```python
from build123d import *

# Parameters (mm, degrees)
SKETCH1_W           = 190.5
SKETCH1_H           = 190.5
SKETCH1_R           = 1.905
SKETCH1_R_2         = 1.778
BOSS_EXTRUDE1_DEPTH = 6.35
BOSS_EXTRUDE3_DEPTH = 6.35
SKETCH8_R           = 3.175
CUT_EXTRUDE1_DEPTH  = 7.35
SKETCH9_R           = 3.175
CUT_EXTRUDE2_DEPTH  = 7.35
SKETCH10_R          = 1.5875
CUT_EXTRUDE3_DEPTH  = 7.35
SKETCH11_R          = 8.41375
CUT_EXTRUDE4_DEPTH  = 7.35


with BuildPart() as part:
    # Sketch1 → Boss-Extrude1 (new body)
    with BuildSketch(Plane(origin=(0, 0, 0), x_dir=(1, 0, 0), z_dir=(0, 1, 0))):
        Rectangle(SKETCH1_W, SKETCH1_H)
        with Locations((-11.303, 11.303)):
            Circle(SKETCH1_R, mode=Mode.SUBTRACT)
        with Locations((-11.303, -11.303)):
            Circle(SKETCH1_R, mode=Mode.SUBTRACT)
        with Locations((11.303, 11.303)):
            Circle(SKETCH1_R, mode=Mode.SUBTRACT)
        with Locations((11.303, -11.303)):
            Circle(SKETCH1_R, mode=Mode.SUBTRACT)
        with Locations((-78.9, 86.55)):
            Circle(SKETCH1_R_2, mode=Mode.SUBTRACT)
        with Locations((-91.6, 86.55)):
            Circle(SKETCH1_R_2, mode=Mode.SUBTRACT)
        with Locations((91.6, -86.55)):
            Circle(SKETCH1_R_2, mode=Mode.SUBTRACT)
        with Locations((78.9, -86.55)):
            Circle(SKETCH1_R_2, mode=Mode.SUBTRACT)
        with Locations((-86.55, -78.9)):
            Circle(SKETCH1_R_2, mode=Mode.SUBTRACT)
        with Locations((-86.55, -91.6)):
            Circle(SKETCH1_R_2, mode=Mode.SUBTRACT)
    extrude(amount=BOSS_EXTRUDE1_DEPTH)

    # Sketch7 → Boss-Extrude3 (add)
    with BuildSketch(Plane.XZ):
        Polygon((-95.25, -130), (78.2, -130), (130, -130), (130, -78.2), (130, 95.25), (95.25, 95.25), (95.25, -95.25), (-95.25, -95.25), align=None)
    extrude(amount=-BOSS_EXTRUDE3_DEPTH)

    # Sketch8 → Cut-Extrude1 (cut, through all)
    with BuildSketch(Plane.XZ):
        with Locations((-63.77864005, -63.77864005)):
            Circle(SKETCH8_R)
        with Locations((-63.77864005, 63.87464005)):
            Circle(SKETCH8_R)
        with Locations((63.87464005, 63.87464005)):
            Circle(SKETCH8_R)
        with Locations((63.87464005, -63.77864005)):
            Circle(SKETCH8_R)
    extrude(amount=-CUT_EXTRUDE1_DEPTH, mode=Mode.SUBTRACT)

    # Sketch9 → Cut-Extrude2 (cut, through all)
    with BuildSketch(Plane.XZ):
        with Locations((123.65, -123.65)):
            Circle(SKETCH9_R)
        with Locations((85.55, -85.55)):
            Circle(SKETCH9_R)
        with Locations((123.65, -85.55)):
            Circle(SKETCH9_R)
        with Locations((85.55, -123.65)):
            Circle(SKETCH9_R)
    extrude(amount=-CUT_EXTRUDE2_DEPTH, mode=Mode.SUBTRACT)

    # Sketch10 → Cut-Extrude3 (cut, through all)
    with BuildSketch(Plane.XZ):
        with Locations((104.6, -123.65)):
            Circle(SKETCH10_R)
        with Locations((85.55, -104.6)):
            Circle(SKETCH10_R)
        with Locations((104.6, -85.55)):
            Circle(SKETCH10_R)
        with Locations((123.65, -104.6)):
            Circle(SKETCH10_R)
    extrude(amount=-CUT_EXTRUDE3_DEPTH, mode=Mode.SUBTRACT)

    # Sketch11 → Cut-Extrude4 (cut, through all)
    with BuildSketch(Plane.XZ):
        with Locations((104.6, -104.6)):
            Circle(SKETCH11_R)
    extrude(amount=-CUT_EXTRUDE4_DEPTH, mode=Mode.SUBTRACT)


solid = part.part
```
Input: part model. Units: mm. Frame: model coordinates. Give positions to 0.01 mm unless a question says otherwise; leave off trailing zeros. Use a Markdown table: item, result.
(1) Pin query (flat end, axial travel): pin 1 (13.5 mm diameter, centred on x = 104.6, z = -104.6, fed in from +Y). Return the tip coordinate at first contact, or that it passes through.
Computed values:
| item | result |
|---|---|
| pin 1 | passes through |
(2) Draft query along X for faces 1 (the cylindrical face through (126.68, 3.13, -84.6)), 2 (the flat face through (-95.25, 3, -16)), 3 (the flat face through (19, 3, 95.25)). Return one class per face: released by +X, released by -X, zero draft, split by the parting line, or undercut.
Computed values:
| item | result |
|---|---|
| face 1 | undercut |
| face 2 | released by -X |
| face 3 | zero draft |
(3) Line query: line 1 (Z direction, x = 104.6, y = 5); line 2 (X direction, y = 3.5, z = 86.55); line 3 (X direction, y = 4.25, z = 78.9). Output: solid intervals per line, ascending. Write a range as from..to.
Computed values:
| item | result |
|---|---|
| line 1 | z = -130..-125.24, -122.06..-113.01, -96.19..-87.14, -83.96..95.25 |
| line 2 | x = -95.25..77.12, 80.68..89.82, 93.38..130 |
| line 3 | x = -95.25..-88.33, -84.77..130 |
